from build123d import *

# Parameters (mm, degrees)
SKETCH1_W               = 30
SKETCH1_H               = 12
SKETCH1_W_2             = 16
SKETCH1_H_2             = 6
BOSS_EXTRUDE1_DEPTH     = 30
FILLET1_R               = 2.5
CUT_EXTRUDE6_DEPTH      = 43.848570571
CUT_EXTRUDE6_DEPTH_BACK = 43.848570571
SKETCH22_R              = 1
SKETCH18_R              = 2.5
SKETCH18_R_2            = 2
SKETCH18_R_3            = 0.85
CUT_EXTRUDE3_DEPTH      = 27
FILLET2_R               = 3
SKETCH23_W              = 3.5
SKETCH23_H              = 20
BOSS_EXTRUDE3_DEPTH     = 7
SKETCH24_R              = 2.5
CUT_EXTRUDE7_DEPTH      = 74
SKETCH19_R              = 4
SKETCH19_R_2            = 1
BOSS_EXTRUDE2_DEPTH     = 20
SKETCH25_R              = 1
CUT_EXTRUDE8_DEPTH      = 4
SKETCH26_R              = 2
CUT_EXTRUDE9_DEPTH      = 1
FILLET3_R               = 10


with BuildPart() as part:
    # Sketch1 → Boss-Extrude1 (new body)
    with BuildSketch(Plane.XY):
        Rectangle(SKETCH1_W, SKETCH1_H)
        Rectangle(SKETCH1_W_2, SKETCH1_H_2, mode=Mode.SUBTRACT)
    extrude(amount=BOSS_EXTRUDE1_DEPTH)

    # Fillet1
    fillet1_edges = [part.edges().sort_by_distance(p)[0] for p in [
        (8, -3, 15),
        (8, 3, 15),
        (-8, 3, 15),
        (-8, -3, 15),
    ]]
    fillet(fillet1_edges, radius=FILLET1_R)

    # Sketch22 → Cut-Extrude6 (cut, two sides: drawn at the far end of the back side and taken through both)
    with BuildSketch(Plane(origin=(15, 0, 0), x_dir=(0, 0, -1), z_dir=(1, 0, 0)).offset(-CUT_EXTRUDE6_DEPTH_BACK)):
        with Locations(Location((-25, 0, 0), (0, 0, 90))):
            Circle(SKETCH22_R)
    extrude(amount=CUT_EXTRUDE6_DEPTH + CUT_EXTRUDE6_DEPTH_BACK, mode=Mode.SUBTRACT)

    # Sketch18 → Cut-Extrude3 (cut)
    with BuildSketch(Plane(origin=(0, 0, 30), x_dir=(-1, 0, 0), z_dir=(0, 0, -1))):
        with Locations((-9.5, 0)):
            Circle(SKETCH18_R)
        with Locations((9.5, 0)):
            Circle(SKETCH18_R)
        Circle(SKETCH18_R_2)
        with Locations((4.5, 0)):
            Circle(SKETCH18_R_3)
        with Locations((-4.5, 0)):
            Circle(SKETCH18_R_3)
    extrude(amount=CUT_EXTRUDE3_DEPTH, mode=Mode.SUBTRACT)

    # Fillet2
    fillet2_edges = [part.edges().sort_by_distance(p)[0] for p in [
        (15, -6, 15),
        (-15, -6, 15),
        (-15, 6, 15),
        (15, 6, 15),
    ]]
    fillet(fillet2_edges, radius=FILLET2_R)

    # Sketch23 → Boss-Extrude3 (add)
    with BuildSketch(Plane(origin=(0, 6, 0), x_dir=(1, 0, 0), z_dir=(0, 1, 0))):
        with Locations((-10.25, -10)):
            Rectangle(SKETCH23_W, SKETCH23_H)
        with Locations((10.25, -10)):
            Rectangle(SKETCH23_W, SKETCH23_H)
    extrude(amount=BOSS_EXTRUDE3_DEPTH)

    # Sketch24 → Cut-Extrude7 (cut)
    with BuildSketch(Plane.ZY.offset(12)):
        with Locations((15, 9.5)):
            Circle(SKETCH24_R)
        with Locations((5, 9.5)):
            Circle(SKETCH24_R)
    extrude(amount=-CUT_EXTRUDE7_DEPTH, mode=Mode.SUBTRACT)

    # Sketch19 → Boss-Extrude2 (add)
    with BuildSketch(Plane(origin=(0, 0, 0), x_dir=(-1, 0, 0), z_dir=(0, 0, -1))):
        with Locations((17.5, 0)):
            Circle(SKETCH19_R)
        with Locations((17.5, 0)):
            Circle(SKETCH19_R_2, mode=Mode.SUBTRACT)
    boss_extrude2 = extrude(amount=-BOSS_EXTRUDE2_DEPTH)

    # Sketch25 → Cut-Extrude8 (cut)
    with BuildSketch(Plane(origin=(-21.5, 0, 0), x_dir=(0, 0, -1), z_dir=(1, 0, 0))):
        with Locations(Location((-10, 0, 0), (0, 0, 180))):
            Circle(SKETCH25_R)
    cut_extrude8 = extrude(amount=CUT_EXTRUDE8_DEPTH, mode=Mode.SUBTRACT)

    # Sketch26 → Cut-Extrude9 (cut)
    with BuildSketch(Plane(origin=(-21.5, 0, 0), x_dir=(0, 0, -1), z_dir=(1, 0, 0))):
        with Locations(Location((-10, 0, 0), (0, 0, 180))):
            Circle(SKETCH26_R)
    cut_extrude9 = extrude(amount=CUT_EXTRUDE9_DEPTH, mode=Mode.SUBTRACT)

    # Mirror1: Boss-Extrude2, Cut-Extrude8, Cut-Extrude9 across plane
    add(boss_extrude2.mirror(Plane(origin=(0, 0, 0), x_dir=(0, 0, 1), z_dir=(1, 0, 0))))
    add(cut_extrude8.mirror(Plane(origin=(0, 0, 0), x_dir=(0, 0, 1), z_dir=(1, 0, 0))), mode=Mode.SUBTRACT)
    add(cut_extrude9.mirror(Plane(origin=(0, 0, 0), x_dir=(0, 0, 1), z_dir=(1, 0, 0))), mode=Mode.SUBTRACT)

    # Fillet3
    fillet3_edges = [part.edges().sort_by_distance(p)[0] for p in [
        (-14.99757668, 3.120557246, 10),
        (-14.99757668, -3.120557246, 10),
        (14.99757668, 3.120557246, 10),
        (14.99757668, -3.120557246, 10),
    ]]
    fillet(fillet3_edges, radius=FILLET3_R)


solid = part.part
The listing builds one solid part. Answer for the finished solid, in the listing's coordinates (mm). A direction names the side the tool comes from. Coordinates: 2 decimals unless noted, no trailing zeros. Loops run counter-clockwise (first coordinate to the right, second up) from the corner with the lowest first, then second, coordinate; pieces in that order, holes last.
1) Find section A-A on x = -3.5. Write down the section's boundary in (y, z), then the cut area to 3 significant figures.
2) Find the intervals of material crossed by L1, parallel to X at y = 6.75, z = 6; L2, parallel to Y at x = -9.5, z = 23.5; L3, parallel to Y at x = 1.5, z = 19.5, in increasing order.
3) Find section B-B on y = 7.5. Write down the section's boundary in (x, z).
4) Flat-ended cylindrical pins translate along their axes: pin 1 Ø2 at (y, z) = (3.5, 19.5) entering from -X; pin 2 Ø3.5 at (y, z) = (0, 10) entering from -X; pin 3 Ø2.5 at (x, y) = (19, -2.5) entering from +Z. Find the tip coordinate at first contact, or state that the pin passes through.
5) Find section D-D on z = 5. Give the number of separate pieces and of enclosed holes in the cut face, then the cut area to 3 significant figures.
6) A tool of negligible diameter and unlimited length cuts with its end or side. For faces 5 (the face through (13.24, 5.73, 18.54)), 6 (the face through (-6.911, 2.564, 15.21)), 7 (the face through (13.298, -5.705, 18.543)), 8 (the face through (-19, 0, 9)), 9 (the face through (-13.24, 5.73, 18.54)), from which of +Z, -Z, +X, -X, +Y, -Y can it reach the whole face along a straight path? Write none if from no direction.
7) Determine the mould class of faces 1 (the face through (0, 4, 0)), 2 (the face through (20.896, -1.686, 11.075)), 3 (the face through (12, 9, 10)), 4 (the face through (10.23, 7.28, 6.15)) for opening direction Z: pulls with the +Z half, pulls with the -Z half, needs draft (parallel to the pull), parting line crosses it, or undercut.
8) Find section C-C on x = 9.5. Write down the section's boundary in (y, z), then the cut area to 3 significant figures.
Values:
1. outline: (-6, 0) - (-3, 0) - (-3, 30) - (-6, 30) - close; (3, 0) - (6, 0) - (6, 30) - (3, 30) - close
1. area: 180 mm2
2. L1: x = -12 to -8.5, 8.5 to 12
2. L2: y = -6 to -2.5, 2.5 to 6
2. L3: y = -6 to -3, 3 to 6
3. outline: (-12, 0) - (-8.5, 0) - (-8.5, 3.5) - (-12, 3.5) - close; (-12, 6.5) - (-8.5, 6.5) - (-8.5, 13.5) - (-12, 13.5) - close; (-12, 16.5) - (-8.5, 16.5) - (-8.5, 20) - (-12, 20) - close; (8.5, 0) - (12, 0) - (12, 3.5) - (8.5, 3.5) - close; (8.5, 6.5) - (12, 6.5) - (12, 13.5) - (8.5, 13.5) - close; (8.5, 16.5) - (12, 16.5) - (12, 20) - (8.5, 20) - close
4. pin 1: stops at x = -20.62
4. pin 2: stops at x = -20.5
4. pin 3: stops at z = 20
5. separate pieces: 3
5. enclosed holes: 3
5. area: 331 mm2
6. face 5: +Z, +X, +Y
6. face 6: +Z, -Z
6. face 7: +Z, +X, -Y
6. face 8: -X
6. face 9: +Z, -X, +Y
7. face 1: pulls with the -Z half
7. face 2: undercut
7. face 3: needs draft
7. face 4: undercut
8. outline: (-6, 0) - (13, 0) - (13, 20) - (6, 20) - (6, 30) - (2.5, 30) - (2.5, 3) - (-2.5, 3) - (-2.5, 30) - (-6, 30) - close; hole circle Ø5 at (9.5, 5); hole circle Ø5 at (9.5, 15)
8. area: 326 mm2
